Source: CAD feature listing. Evaluate the final solid. Frame: model axes, mm. Face numbers are marked on the shaded views. A direction names the side the tool comes from. Coordinates: 2 decimals unless noted, no trailing zeros. Order: outer loops, then holes, each group sorted by start corner. A loop starts at its lowest first (then second) coordinate and runs counter-clockwise, first axis right, second up.
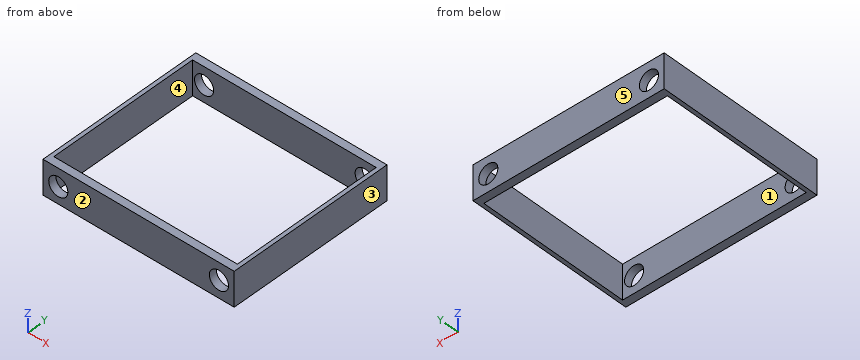
Autodesk Inventor part; units mm, degrees
ref_plane "YZ Plane" through (0, 0, 0) normal (1, 0, 0) x (0, 1, 0)
ref_plane "XZ Plane" through (0, 0, 0) normal (0, 1, 0) x (-1, 0, 0)
ref_plane "XY Plane" through (0, 0, 0) normal (0, 0, 1) x (1, 0, 0)
sketch "Sketch1" plane through (0, 0, 0) normal (0, 0, 1) x (1, 0, 0)
  line L0 (0, 0) -> (0, 43.57)
  line L1 (0, 43.57) -> (50, 43.57)
  line L2 (50, 43.57) -> (50, 0)
  line L3 (50, 0) -> (0, 0)
  line L4 (1, 1) -> (1, 42.57)
  line L5 (1, 42.57) -> (49, 42.57)
  line L6 (49, 42.57) -> (49, 1)
  line L7 (49, 1) -> (1, 1)
  dimension "d0" = 43.57
  dimension "d1" = 50
  dimension "d2" = 41.57
  dimension "d3" = 48
extrude "Extrusion1" add sketch "Sketch1" along normal blind 9
sketch "Sketch2" plane through (1, 42.57, 0) normal (0, -1, 0) x (1, 0, 0)
  line L0 (48, 0) -> (0, 0)
  line L1 (48, 0) -> (48, 9)
  line L2 (0, 9) -> (48, 9)
  line L3 (0, 0) -> (0, 9)
  point P0 (-1, 0)
extrude "Extrusion2" add sketch "Sketch2" along normal blind 1
sketch "Sketch3" plane through (1, 1, 0) normal (0, 1, 0) x (1, 0, 0)
  line L0 (0, 0) -> (48, 0)
  line L1 (0, 0) -> (0, -9)
  line L2 (48, -9) -> (0, -9)
  line L3 (48, 0) -> (48, -9)
  point P0 (-1, 0)
extrude "Extrusion3" add sketch "Sketch3" along normal blind 1
sketch "Sketch4" plane through (0, 43.57, 0) normal (0, 1, 0) x (1, 0, 0)
  point P0 (4, -4.3741)
  point P1 (46, -4.5)
hole "Hole1" at (4, 43.57, 4.3741) at (46, 43.57, 4.5) direction (0, -1, 0) diameter 5 end through all
properties part number "Hoofdplaat zijkant"
1. Section query C-C on z = 1. Return loops of the section in (x, y), plus the area to 3 significant figures.
Findings:
outline: (0, 0) - (50, 0) - (50, 43.57) - (0, 43.57) - close; hole (1, 2) - (49, 2) - (49, 41.57) - (1, 41.57) - close
area: 279 mm2
2. Draft query along X for the marked faces 1, 2 and 3. Return one class per face: released by +X, released by -X, zero draft, split by the parting line, or undercut.
Findings:
face 1: undercut
face 2: zero draft
face 3: released by +X
3. Ray query, line 1 (X direction, y = 42.1, z = 4.5); line 2 (Z direction, x = 46, y = 1.55); line 3 (Y direction, x = 36, z = 6.25). Return the intervals inside material, ascending.
Findings:
line 1: x = 0 to 1.5, 6.5 to 43.5, 48.5 to 50
line 2: z = 0 to 2, 7 to 9
line 3: y = 0 to 2, 41.57 to 43.57
4. Section query D-D on x = 41. Return loops of the section in (y, z), plus the area to 3 significant figures.
Findings:
outline: (0, 0) - (2, 0) - (2, 9) - (0, 9) - close; (41.57, 0) - (43.57, 0) - (43.57, 9) - (41.57, 9) - close
area: 36.0 mm2
5. Access query for the marked faces 4 and 5. Directions: +Z, -Z, +X, -X, +Y, -Y. A direction counts if a zero-diameter tool reaches every point of the face in a straight line with its end or side. Return the directions, or none.
Findings:
face 4: +Z, -Z
face 5: +Z, -Z, +X, -X, +Y
6. Section query B-B on y = 32.5. Return loops of the section in (x, z), plus the area to 3 significant figures.
Findings:
outline: (0, 0) - (1, 0) - (1, 9) - (0, 9) - close; (49, 0) - (50, 0) - (50, 9) - (49, 9) - close
area: 18.0 mm2
7. Section query A-A on x = 46. Return loops of the section in (y, z), plus the area to 3 significant figures.
Findings:
outline: (0, 0) - (2, 0) - (2, 2) - (0, 2) - close; (0, 7) - (2, 7) - (2, 9) - (0, 9) - close; (41.57, 0) - (43.57, 0) - (43.57, 2) - (41.57, 2) - close; (41.57, 7) - (43.57, 7) - (43.57, 9) - (41.57, 9) - close
area: 16.0 mm2
